Can you work these out from the model? Positions are in its coordinate system, mm. Face numbers are marked on the shaded views. A direction names the side the tool comes from. Coordinates: 2 decimals unless noted, no trailing zeros. Loops run counter-clockwise (first coordinate to the right, second up) from the corner with the lowest first, then second, coordinate; pieces in that order, holes last. Notation, with made-up numbers: M 58,-8.5 L 84,-8.5 A17 cw 84,4.5 Z; hole C 80,48 d7. An arc over 180 degrees is marked long. Answer as a JSON object with one key per item and string values. Group by question number.
Item 1: Which directions (+Z, -Z, +X, -X, +Y, -Y) give clear straight access to the entire face, cutting with the end or side of a thin tool? Please do the marked faces 5, 6, 7, 8 and 9.
Item 2: Suppose I cut it at D-D (z = 21). Write out the boundary of the cut face in (x, y).
Item 3: Suppose I cut it at C-C (x = -1). Write out the boundary of the cut face in (y, z), then the cut area to 3 significant figures.
Item 4: Suppose I cut it at B-B (y = -22). Write out the boundary of the cut face in (x, z), then the cut area to 3 significant figures.
Item 5: If I drill on line 1 (X direction, y = -43, z = -6); line 2 (Z direction, x = -1, y = -36); line 3 (X direction, y = -47, z = -8), over which ranges is the centre line in solid material (lowest first)?
Item 6: We'd pull the mould along X, two halves only. Please class the marked faces 1, 2, 3 and 4: +X half, -X half, draft (parallel to the pull), parting line (faces both ways), or undercut.
Item 7: Suppose I cut it at A-A (z = -2). Write out the boundary of the cut face in (x, y), then the cut area to 3 significant figures.
Item 8: I'm going to push flat-ended pins straight in: pin 1 Ø3.5 at (y, z) = (-42.5, -6) entering from -X; pin 2 Ø1 at (x, y) = (11.5, 30.5) entering from -Z; pin 3 Ø8.5 at (x, z) = (42.5, -3) entering from -Y. Where does each tip first touch, or does it pass through?
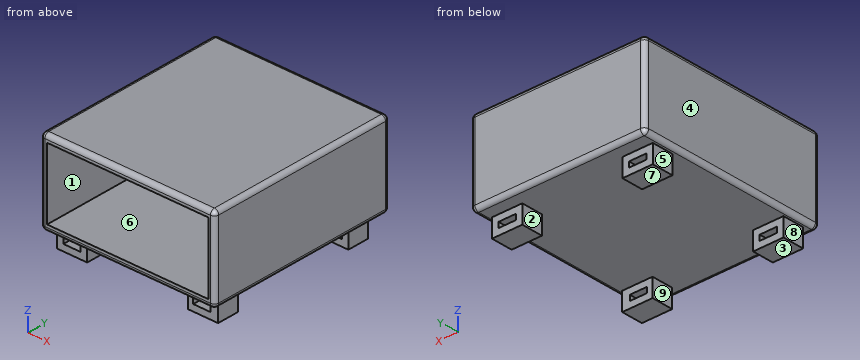
```python
from build123d import *

# Parameters (mm, degrees)
F0_W      = 102.235
F0_H      = 109.855
F1_DEPTH  = 49.53
F2_W      = 94.615
F2_H      = 41.275
F3_DEPTH  = 111.252
F4_W      = 17.78
F4_H      = 12.7
F5_DEPTH  = 10.795
F6_W      = 10.16
F6_H      = 3.175
F7_DEPTH  = 12.7
F8_W      = 102.235
F8_H      = 49.53
F9_DEPTH  = 3.048
F10_W     = 10.16
F10_H     = 3.175
F11_DEPTH = 25.4
F12_W     = 10.16
F12_H     = 3.175
F13_DEPTH = 25.4
F14_R     = 2.54
F15_W     = 10.16
F15_H     = 3.175
F16_DEPTH = 25.4
F17_W     = 10.16
F17_H     = 3.175
F18_DEPTH = 25.4


with BuildPart() as f1:
    # F0 (on Top) → F1 (new body)
    with BuildSketch(Plane.XY):
        Rectangle(F0_W, F0_H)
    extrude(amount=F1_DEPTH)

    # F2 (on face) → F3 (cut)
    with BuildSketch(Plane.XZ.offset(54.9275)):
        with Locations((0, 24.765)):
            Rectangle(F2_W, F2_H)
    extrude(amount=-F3_DEPTH, mode=Mode.SUBTRACT)

    # F4 (on face) → F5 (join)
    with BuildSketch(Plane(origin=(0, 0, 0), x_dir=(1, 0, 0), z_dir=(0, 0, -1))):
        with Locations((-38.290499, -42.132252)):
            Rectangle(F4_W, F4_H)
        Polygon((-38.4175, 48.5775), (-47.3075, 48.5775), (-47.3075, 35.8775), (-29.5275, 35.8775), (-29.5275, 48.5775), align=None)
        Polygon((47.3075, 48.5775), (38.4175, 48.5775), (29.5275, 48.5775), (29.5275, 35.8775), (47.3075, 35.8775), align=None)
        Polygon((29.400499, -48.482252), (38.4175, -48.482252), (47.180499, -48.482252), (47.180499, -35.782252), (29.400499, -35.782252), align=None)
    extrude(amount=F5_DEPTH)

    # F6 (on face) → F7 (cut)
    with BuildSketch(Plane(origin=(-51.1175, 0, 0), x_dir=(0, -1, 0), z_dir=(-1, 0, 0))):
        with Locations((-26.9875, -3.175)):
            Rectangle(F6_W, F6_H)
        with Locations((26.9875, -3.175)):
            Rectangle(F6_W, F6_H)
    extrude(amount=-F7_DEPTH, mode=Mode.SUBTRACT)

    # F8 (on face) → F9 (join)
    with BuildSketch(Plane(origin=(0, 54.9275, 0), x_dir=(-1, 0, 0), z_dir=(0, 1, 0))):
        with Locations((0, 24.765)):
            Rectangle(F8_W, F8_H)
    extrude(amount=F9_DEPTH)

    # F10 (on face) → F11 (cut)
    with BuildSketch(Plane.XZ.offset(48.5775)):
        with Locations((-38.4175, -5.3975)):
            Rectangle(F10_W, F10_H)
    extrude(amount=-F11_DEPTH, mode=Mode.SUBTRACT)

    # F12 (on face) → F13 (cut)
    with BuildSketch(Plane.XZ.offset(-35.782252)):
        with Locations((-38.290499, -5.3975)):
            Rectangle(F12_W, F12_H)
    extrude(amount=-F13_DEPTH, mode=Mode.SUBTRACT)

    # F14
    f14_edges = [f1.edges().sort_by_distance(p)[0] for p in [
        (-51.1175, -54.9275, 24.765),
        (51.1175, -54.9275, 24.765),
        (51.1175, 57.9755, 24.765),
        (-51.1175, 57.9755, 24.765),
        (0, 57.9755, 0),
        (51.1175, 1.524, 0),
        (51.1175, 1.524, 49.53),
        (-51.1175, 1.524, 0),
        (-51.1175, 1.524, 49.53),
        (0, 57.9755, 49.53),
        (0, -54.9275, 49.53),
        (0, -54.9275, 0),
    ]]
    fillet(f14_edges, radius=F14_R)

    # F15 (on face) → F16 (cut)
    with BuildSketch(Plane(origin=(0, 48.482252, 0), x_dir=(-1, 0, 0), z_dir=(0, 1, 0))):
        with Locations((-38.290499, -5.3975)):
            Rectangle(F15_W, F15_H)
    extrude(amount=-F16_DEPTH, mode=Mode.SUBTRACT)

    # F17 (on face) → F18 (cut)
    with BuildSketch(Plane(origin=(0, -35.8775, 0), x_dir=(-1, 0, 0), z_dir=(0, 1, 0))):
        with Locations((-37.7825, -5.3975)):
            Rectangle(F17_W, F17_H)
    extrude(amount=-F18_DEPTH, mode=Mode.SUBTRACT)


solid = f1.part
```
From the geometry:
{
 "1": {"face 5": "-Z, -X, +Y", "face 6": "-Y", "face 7": "-Z, +X, -X, +Y, -Y", "face 8": "-Z, -X, +Y, -Y", "face 9": "-Z, -Y"},
 "2": {"outline": "M -51.12,-52.39 A2.54 ccw -48.58,-54.93 L -47.31,-54.93 L -47.31,54.93 L 47.31,54.93 L 47.31,-54.93 L 48.58,-54.93 A2.54 ccw 51.12,-52.39 L 51.12,55.44 A2.54 ccw 48.58,57.98 L -48.58,57.98 A2.54 ccw -51.12,55.44 Z"},
 "3": {"outline": "M -54.93,2.54 A2.54 ccw -52.39,0 L 55.44,0 A2.54 ccw 57.98,2.54 L 57.98,46.99 A2.54 ccw 55.44,49.53 L -52.39,49.53 A2.54 ccw -54.93,46.99 L -54.93,45.4 L 54.93,45.4 L 54.93,4.13 L -54.93,4.13 Z", "area": "1,050 mm2"},
 "4": {"outline": "M -51.12,2.54 A2.54 ccw -48.58,0 L 48.58,0 A2.54 ccw 51.12,2.54 L 51.12,46.99 A2.54 ccw 48.58,49.53 L -48.58,49.53 A2.54 ccw -51.12,46.99 Z; hole M -47.31,4.13 L 47.31,4.13 L 47.31,45.4 L -47.31,45.4 Z", "area": "1,150 mm2"},
 "5": {"line 1": "-47.31 to -43.5, -33.34 to -29.53, 29.53 to 32.7, 42.86 to 47.31", "line 2": "0 to 4.13, 45.4 to 49.53", "line 3": "-47.31 to -29.53, 29.53 to 47.31"},
 "6": {"face 1": "undercut", "face 2": "undercut", "face 3": "draft", "face 4": "-X half"},
 "7": {"outline": "M -47.31,-48.58 L -29.53,-48.58 L -29.53,-35.88 L -47.31,-35.88 Z; M -47.18,35.78 L -29.4,35.78 L -29.4,48.48 L -47.18,48.48 Z; M 29.4,35.78 L 47.18,35.78 L 47.18,48.48 L 29.4,48.48 Z; M 29.53,-48.58 L 47.31,-48.58 L 47.31,-35.88 L 29.53,-35.88 Z", "area": "903 mm2"},
 "8": {"pin 1": "x = -47.31", "pin 2": "z = 0", "pin 3": "y = -54.58"}
}
